Source: CAD feature listing. Evaluate the final solid. Frame: model axes, mm. Give positions to 0.01 mm unless a question says otherwise; leave off trailing zeros. Order: outer loops, then holes, each group sorted by start corner. A loop starts at its lowest first (then second) coordinate and runs counter-clockwise, first axis right, second up. Notation, with made-up numbers: (18, 37) - (63, 37) arc R36 cw to (63, 72) - close; hole circle Ø8 at (38, 62.5). An arc over 180 degrees is marked (long way). Use CSV: the item, a comma, the result in double quotes.
```python
from build123d import *

# Parameters (mm, degrees)
F1_DEPTH = 6.35


# Not quite as in the source:
# - a feature names something its author has since deleted; it is built from what else it names


with BuildPart() as f1:
    # F0 (on Top) → F1 (new body)
    with BuildSketch(Plane.XY):
        with BuildLine():
            ThreePointArc((-20.6136406437, -48.4949748961), (-18.1522527003, -49.6160033902), (-15.474999986, -50))
            ThreePointArc((-15.474999986, -50), (-11.7658348983, -49.248124828), (-8.64225073, -47.1112009021))
            ThreePointArc((-8.64225073, -47.1112009021), (-0.3913128261, -49.2725077899), (8.1069210399, -50))
            ThreePointArc((8.1069210399, -50), (58.1069208781, 4.4e-08), (8.1069209519, 50))
            ThreePointArc((8.1069209519, 50), (-0.3913128695, 49.2725077824), (-8.64225073, 47.1112009021))
            ThreePointArc((-8.64225073, 47.1112009021), (-11.7658349048, 49.2481248308), (-15.475, 50))
            ThreePointArc((-15.475, 50), (-17.9163659919, 49.6818103648), (-20.1946207283, 48.7485001771))
            ThreePointArc((-20.1946207283, 48.7485001771), (-23.7115044996, 45.2588915778), (-25, 40.4749999628))
            ThreePointArc((-25, 40.4749999628), (-24.7547421233, 38.3274406584), (-24.0315987301, 36.2904757532))
            ThreePointArc((-24.0315987301, 36.2904757532), (-21.6846733781, 33.2524255603), (-18.3290256128, 31.3876371921))
            ThreePointArc((-18.3290256128, 31.3876371921), (-5.6085763504, -0.3160997755), (-19.1387594108, -31.6828164271))
            ThreePointArc((-19.1387594108, -31.6828164271), (-21.6396911965, -33.2139940469), (-23.5563206429, -35.433385014))
            ThreePointArc((-23.5563206429, -35.433385014), (-24.6319701355, -37.8528781611), (-25, -40.475))
            ThreePointArc((-25, -40.475), (-23.8317690267, -45.0455619386), (-20.6136406437, -48.4949748961))
        make_face()
    extrude(amount=F1_DEPTH)


solid = f1.part
```
Item 1: Section B-B on x = 29. Return the cut outline in (y, z), then the cut area to 3 significant figures.
Filled in:
outline,"(-45.43, 0) - (45.43, 0) - (45.43, 6.35) - (-45.43, 6.35) - close"
area,"577 mm2"
Item 2: First-contact query: pin 1 (1.5 mm diameter, centred on y = -0.5, z = 1, fed in from +X). Flat tip, straight axial feed; report the tip coordinate or a pass-through.
Filled in:
pin 1,"stops at x = 58.11"
Item 3: Section C-C on y = 11.5. Return the cut outline in (x, z).
Filled in:
outline,"(-7.05, 0) - (56.77, 0) - (56.77, 6.35) - (-7.05, 6.35) - close"
Item 4: Material intervals for line 1 (Y direction, x = 37.5, z = 3.5); line 2 (Y direction, x = -21.5, z = 0.5); line 3 (Y direction, x = -9.5, z = 2), sorted ascending. Write a range as from..to.
Filled in:
line 1,"y = -40.45..40.45"
line 2,"y = -47.85..-33.1, 33.1..47.85"
line 3,"y = -47.89..-17.94, 18.45..47.89"
Item 5: Mould query, pull axis Y, two halves, no side actions, for faces 1 (the flat face through (16, 1, 0)), 2 (the cylindrical face through (-5.605, 0.175, 3.131)). Classes: released by +Y, released by -Y, zero draft, split by the parting line, or undercut.
Filled in:
face 1,"zero draft"
face 2,"undercut"
